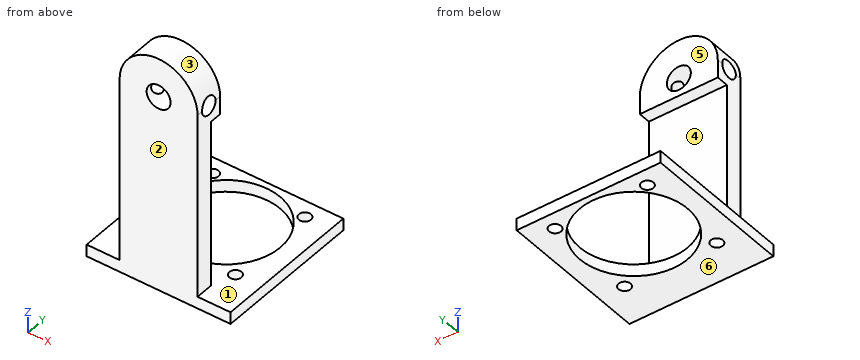
from build123d import *

# Parameters (mm, degrees)
SKETCH_2_R               = 6.5
EXTRUDE_1_DEPTH          = 5
SKETCH_3_R               = 2
CUT_EXTRUDE_2_DEPTH      = 11.464224768
EXTRUDE_START            = -5
EXTRUDE_2_DEPTH          = 5
EXTRUDE_3_DEPTH          = 2
SKETCH_22_R              = 9
SKETCH_22_R_2            = 1
CUT_EXTRUDE_4_DEPTH      = 2
CUT_EXTRUDE_6_DEPTH      = 44.104524125
CUT_EXTRUDE_6_DEPTH_BACK = 44.104524125
SKETCH_23_R              = 1.5
SKETCH_24_W              = 13
SKETCH_24_H              = 28
CUT_EXTRUDE_7_DEPTH      = 2


with BuildPart() as part:
    # 草图2 → 凸台-拉伸1 (new body)
    with BuildSketch(Plane(origin=(0, 0, 0), x_dir=(1, 0, 0), z_dir=(0, 1, 0))):
        with Locations(Location((0, 0, 0), (0, 0, 270))):
            Circle(SKETCH_2_R)
    extrude(amount=EXTRUDE_1_DEPTH)

    # 草图3 → 切除-拉伸2 (cut, through all)
    with BuildSketch(Plane(origin=(0, 5, 0), x_dir=(1, 0, 0), z_dir=(0, 1, 0))):
        with Locations(Location((0, 0, 0), (0, 0, 270))):
            Circle(SKETCH_3_R)
    extrude(amount=-CUT_EXTRUDE_2_DEPTH, mode=Mode.SUBTRACT)

    # 草图4 → 凸台-拉伸2 (add)
    with BuildSketch(Plane(origin=(0, 5, 0), x_dir=(1, 0, 0), z_dir=(0, 1, 0)).offset(EXTRUDE_START)):
        with BuildLine():
            Line((6.5, 0), (6.5, 31))
            Line((6.5, 31), (3.899148682, 31))
            Line((3.899148682, 31), (-4.100851318, 31))
            Line((-4.100851318, 31), (-6.5, 31))
            Line((-6.5, 31), (-6.5, 0))
            ThreePointArc((-6.5, 0), (0, 6.5), (6.5, 0))
        make_face()
    extrude(amount=EXTRUDE_2_DEPTH)

    # 草图21 → 凸台-拉伸3 (add)
    with BuildSketch(Plane(origin=(0, 0, -31), x_dir=(-1, 0, 0), z_dir=(0, 0, -1))):
        Polygon((0, 0), (12, 0), (12, 25), (-12, 25), (-12, 0), align=None)
    extrude(amount=EXTRUDE_3_DEPTH)

    # 草图22 → 切除-拉伸4 (cut)
    with BuildSketch(Plane.XY.offset(-31)):
        with Locations((0, 15)):
            Circle(SKETCH_22_R)
        with Locations((7.7, 22.2)):
            Circle(SKETCH_22_R_2)
        with Locations((-7.7, 22.2)):
            Circle(SKETCH_22_R_2)
        with Locations((-7.7, 6.8)):
            Circle(SKETCH_22_R_2)
        with Locations((7.7, 6.8)):
            Circle(SKETCH_22_R_2)
    extrude(amount=-CUT_EXTRUDE_4_DEPTH, mode=Mode.SUBTRACT)

    # 草图23 → 切除-拉伸6 (cut, two sides: drawn at the far end of the back side and taken through both)
    with BuildSketch(Plane(origin=(0, 0, 0), x_dir=(0, 0, -1), z_dir=(1, 0, 0)).offset(-CUT_EXTRUDE_6_DEPTH_BACK)):
        with Locations((0, 2.5)):
            Circle(SKETCH_23_R)
    extrude(amount=CUT_EXTRUDE_6_DEPTH + CUT_EXTRUDE_6_DEPTH_BACK, mode=Mode.SUBTRACT)

    # 草图24 → 切除-拉伸7 (cut)
    with BuildSketch(Plane(origin=(0, 5, 0), x_dir=(1, 0, 0), z_dir=(0, 1, 0))):
        with Locations((0, 17)):
            Rectangle(SKETCH_24_W, SKETCH_24_H)
    extrude(amount=-CUT_EXTRUDE_7_DEPTH, mode=Mode.SUBTRACT)


solid = part.part
CAD build for the part. Positions are in the model's coordinates, mm. Face numbers are marked on the shaded views. A direction names the side the tool comes from. Give positions to 0.01 mm unless a question says otherwise; leave off trailing zeros. Loops run counter-clockwise (first coordinate to the right, second up) from the corner with the lowest first, then second, coordinate; pieces in that order, holes last. Notation, with made-up numbers: M -0.75,62 L 29.25,62 A32 ccw 29.25,88 Z; hole C -26,-15 d11. An arc over 180 degrees is marked long. Answer in a Markdown table with one row per item. Add a question column.
Item 1: Drop flat-ended pins along their axis: P1, Ø4, axis at y = 3, z = -15.5, coming from the -X side; P2, Ø3, axis at x = -7.7, y = 22.2, coming from the +Z side; P3, Ø10, axis at x = -7, y = 6, coming from the +Z side. Give the stop position or say it passes through.
Item 2: Band-saw the part on D-D on y = 12. Give the cut face in (x, z), then the cut area to 3 significant figures.
Item 3: Probe probe 1 along Y at (x, z) = (7.7, -31.9); probe 2 along X at (y, z) = (1.75, -19); probe 3 along Z at (x, y) = (-2.5, 2.5). List the from-to ranges inside material, lowest first.
Item 4: Tool access for the marked faces 4, 5 and 6: list every direction of +Z, -Z, +X, -X, +Y, -Y with a clear straight run to the whole face (end or side of a thin tool).
Item 5: Band-saw the part on C-C on x = 7.7. Give the cut face in (y, z), then the cut area to 3 significant figures.
Item 6: Mould opens along Z. For the marked faces 1, 2 and 3 say: +Z half, -Z half, draft (parallel to the pull), parting line (faces both ways), or undercut.
Item 7: Band-saw the part on A-A on y = 22.2. Give the cut face in (x, z), then the cut area to 3 significant figures.
Item 8: Band-saw the part on B-B on x = -3. Give the cut face in (y, z), then the cut area to 3 significant figures.
Reply:
| question | item | result |
|---|---|---|
| 1 | P1 | stops at x = -6.5 |
| 1 | P2 | stops at z = -31 |
| 1 | P3 | stops at z = 6.15 |
| 2 | outline | M -12,-33 L -8.49,-33 L -8.49,-31 L -12,-31 Z; M 8.49,-33 L 12,-33 L 12,-31 L 8.49,-31 Z |
| 2 | area | 14.1 mm^2 |
| 3 | probe 1 | y = 0 to 5.8, 7.8 to 10.34, 19.66 to 21.2, 23.2 to 25 |
| 3 | probe 2 | x = -6.5 to 6.5 |
| 3 | probe 3 | z = -33 to -1.5, 1.5 to 6 |
| 4 | face 4 | +X, -X, +Y |
| 4 | face 5 | +Z, +X, -X, +Y |
| 4 | face 6 | -Z, +X, -X, +Y, -Y |
| 5 | outline | M 0,-33 L 5.8,-33 L 5.8,-31 L 0,-31 Z; M 7.8,-33 L 10.34,-33 L 10.34,-31 L 7.8,-31 Z; M 19.66,-33 L 21.2,-33 L 21.2,-31 L 19.66,-31 Z; M 23.2,-33 L 25,-33 L 25,-31 L 23.2,-31 Z |
| 5 | area | 23.4 mm^2 |
| 6 | face 1 | undercut |
| 6 | face 2 | draft |
| 6 | face 3 | +Z half |
| 7 | outline | M -12,-33 L -8.7,-33 L -8.7,-31 L -12,-31 Z; M -6.7,-33 L -5.4,-33 L -5.4,-31 L -6.7,-31 Z; M 5.4,-33 L 6.7,-33 L 6.7,-31 L 5.4,-31 Z; M 8.7,-33 L 12,-33 L 12,-31 L 8.7,-31 Z |
| 7 | area | 18.4 mm^2 |
| 8 | outline | M 0,-33 L 6.51,-33 L 6.51,-31 L 3,-31 L 3,-3 L 5,-3 L 5,5.77 L 0,5.77 Z; M 23.49,-33 L 25,-33 L 25,-31 L 23.49,-31 Z; hole C 2.5,0 d3 |
| 8 | area | 137 mm^2 |
